Study the drawing (mm; zero at the part's minimum x, y, z) and answer. Coordinates: 2 decimals unless noted, no trailing zeros. Loops run counter-clockwise (first coordinate to the right, second up) from the corner with the lowest first, then second, coordinate; pieces in that order, holes last. Notation, with made-up numbers: (-29.5, 85.5) -> (6.5, 85.5) arc R22 ccw to (6.5, 105.5) -> close; hole circle Ø9 at (-11.5, 24.25). An arc over 180 degrees is marked (long way). Answer in a Markdown table with one row per item.
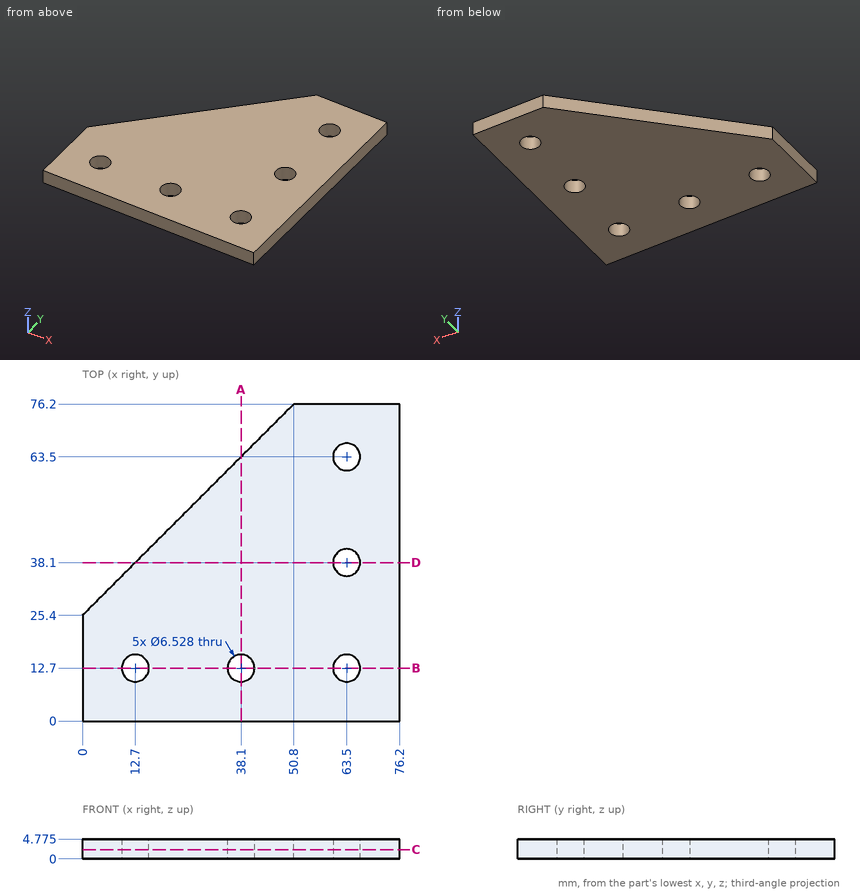
1. A cutting plane is placed at A-A on x = 38.1. Give the vertices of the cut face in (y, z) (1 decimal).
A:
| item | result |
|---|---|
| outline | (0, 0) -> (9.4, 0) -> (9.4, 4.8) -> (0, 4.8) -> close; (16, 0) -> (63.5, 0) -> (63.5, 4.8) -> (16, 4.8) -> close |
2. Given pin 1 Ø8.5 at (x, y) = (38.1, 12.7) entering from -Z; pin 2 Ø1 at (x, z) = (27, 2) entering from +Y; pin 3 Ø1.5 at (x, z) = (31, 0.5) entering from +Y, each flat-ended and moving along its own axis, determine where each tip first touches the part or whether it passes through.
A:
| item | result |
|---|---|
| pin 1 | stops at z = 0 |
| pin 2 | stops at y = 52.9 |
| pin 3 | stops at y = 57.15 |
3. Find the intervals of material crossed by probe 1 along Y at (x, z) = (63.5, 2.1); probe 2 along Y at (x, z) = (64.5, 1.5); probe 3 along Y at (x, z) = (38.1, 3.6) (1 decimal), in increasing order.
A:
| item | result |
|---|---|
| probe 1 | y = 0 to 9.44, 15.96 to 34.84, 41.36 to 60.24, 66.76 to 76.2 |
| probe 2 | y = 0 to 9.59, 15.81 to 34.99, 41.21 to 60.39, 66.61 to 76.2 |
| probe 3 | y = 0 to 9.4, 16 to 63.5 |
4. A cutting plane is placed at D-D on y = 38.1. Give the vertices of the cut face in (x, z) (1 decimal), and give its area (3 significant figures).
A:
| item | result |
|---|---|
| outline | (12.7, 0) -> (60.2, 0) -> (60.2, 4.8) -> (12.7, 4.8) -> close; (66.8, 0) -> (76.2, 0) -> (76.2, 4.8) -> (66.8, 4.8) -> close |
| area | 272 mm2 |
5. A cutting plane is placed at C-C on z = 2.2. Give the vertices of the cut face in (x, y).
A:
| item | result |
|---|---|
| outline | (0, 0) -> (76.2, 0) -> (76.2, 76.2) -> (50.8, 76.2) -> (0, 25.4) -> close; hole circle Ø6.53 at (12.7, 12.7); hole circle Ø6.53 at (38.1, 12.7); hole circle Ø6.53 at (63.5, 12.7); hole circle Ø6.53 at (63.5, 38.1); hole circle Ø6.53 at (63.5, 63.5) |
6. A cutting plane is placed at B-B on y = 12.7. Give the vertices of the cut face in (x, z) (1 decimal), and give its area (3 significant figures).
A:
| item | result |
|---|---|
| outline | (0, 0) -> (9.4, 0) -> (9.4, 4.8) -> (0, 4.8) -> close; (16, 0) -> (34.8, 0) -> (34.8, 4.8) -> (16, 4.8) -> close; (41.4, 0) -> (60.2, 0) -> (60.2, 4.8) -> (41.4, 4.8) -> close; (66.8, 0) -> (76.2, 0) -> (76.2, 4.8) -> (66.8, 4.8) -> close |
| area | 270 mm2 |
